```python
from build123d import *

# Parameters (mm, degrees)
F0_W     = 3
F0_H     = 15
F1_DEPTH = 16
F0_W_2   = 12
F2_DEPTH = 3
F3_R     = 5.5
F4_DEPTH = 1
F5_SIZE  = 2
F6_R     = 5
F7_R     = 0.5


with BuildPart() as f1:
    # F0 (on Top) → F1 (new body)
    with BuildSketch(Plane.XY):
        with Locations((-6, 0)):
            Rectangle(F0_W, F0_H)
    extrude(amount=F1_DEPTH)

    # F0 (on Top) → F2 (join)
    with BuildSketch(Plane.XY):
        with Locations((1.5, 0)):
            Rectangle(F0_W_2, F0_H)
        with BuildLine():
            ThreePointArc((0, -1), (-1, 0), (0, 1))
            Line((0, 1), (2, 1))
            ThreePointArc((2, 1), (2.7071067812, 0.7071067812), (3, 0))
            ThreePointArc((3, 0), (2.7071067812, -0.7071067812), (2, -1))
            Line((2, -1), (0, -1))
        make_face(mode=Mode.SUBTRACT)
    extrude(amount=F2_DEPTH)

    # F3 (on face) → F4 (cut)
    with BuildSketch(Plane(origin=(-7.5, 0, 0), x_dir=(0, -1, 0), z_dir=(-1, 0, 0))):
        with Locations((0, 8)):
            Circle(F3_R)
    extrude(amount=-F4_DEPTH, mode=Mode.SUBTRACT)

    # F5
    f5_edges = [f1.edges().sort_by_distance(p)[0] for p in [
        (-1, 0, 3),
    ]]
    chamfer(f5_edges, length=F5_SIZE)

    # F6
    f6_edges = [f1.edges().sort_by_distance(p)[0] for p in [
        (-6, -7.5, 16),
        (-6, 7.5, 16),
        (7.5, -7.5, 1.5),
        (7.5, 7.5, 1.5),
    ]]
    fillet(f6_edges, radius=F6_R)

    # F7
    f7_edges = [f1.edges().sort_by_distance(p)[0] for p in [
        (-7.5, 5.5, 8),
        (-7.5, 6.035534, 14.535534),
        (-4.5, -6.035534, 14.535534),
        (6.035534, -6.035534, 3),
    ]]
    fillet(f7_edges, radius=F7_R)


solid = f1.part
```
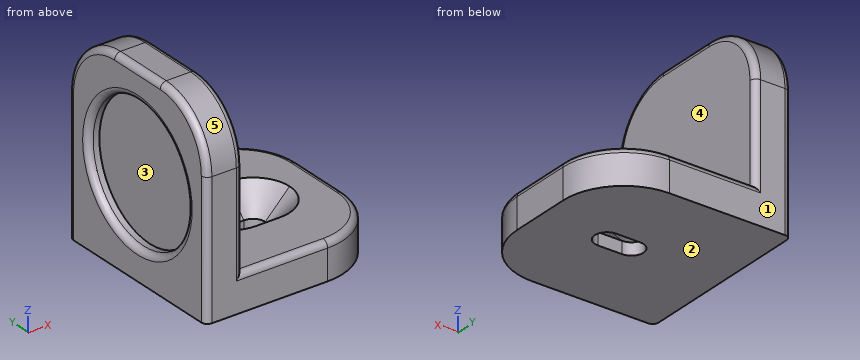
Design review of the part built by this model. Coordinates are the model's own, in mm. Face numbers are marked on the shaded views. A direction names the side the tool comes from. Coordinates: 2 decimals unless noted, no trailing zeros. Order: outer loops, then holes, each group sorted by start corner. A loop starts at its lowest first (then second) coordinate and runs counter-clockwise, first axis right, second up.
1) Take a section at A-A, the plane x = 1.25. Give the boundary of the cut face in (y, z), and give its area (3 significant figures).
2) Mouldability with a two-part tool opening along Z and no side actions: class the marked faces 1, 2 and 3 as +Z half, -Z half, draft (parallel to the pull), parting line (faces both ways), or undercut.
3) Wall thickness on line 1 along Z through (x, y) = (-6.7, 0); line 2 along Z through (x, y) = (5.5, 3.5); line 3 along X through (y, z) = (6.5, 6): over which ranges is each line inside the solid? List them lowest first.
4) For the marked faces 4 and 5, list the 3-axis set-ups (+Z, -Z, +X, -X, +Y, -Y) from which the entire face can be reached by the end or side of a thin tool; tool diameter is ignored.
5) Clearance check with flat-ended pins moving along their axes: pin 1 (4 mm diameter, centred on y = 3, z = 11.5, fed in from +X); pin 2 (6 mm diameter, centred on x = -3.5, z = 6, fed in from +Y); pin 3 (9 mm diameter, centred on x = 2.5, y = -2.5, fed in from +Z). State where each tip first meets the part, or that it passes through.
6) Take a section at B-B, the plane z = 8. Give the boundary of the cut face in (x, y).
Returned:
1. outline: (-7.5, 0) - (-1, 0) - (-1, 1) - (-3, 3) - (-7, 3) arc R0.5 ccw to (-7.5, 2.5) - close; (1, 0) - (7.5, 0) - (7.5, 2.5) arc R0.5 ccw to (7, 3) - (3, 3) - (1, 1) - close
1. area: 34.9 mm2
2. face 1: draft
2. face 2: -Z half
2. face 3: undercut
3. line 1: z = 0 to 2.5, 13.5 to 16
3. line 2: z = 0 to 3
3. line 3: x = -7.5 to -4.5
4. face 4: +Z, +X, +Y, -Y
4. face 5: +Z, +X, -X, -Y
5. pin 1: stops at x = -4.5
5. pin 2: stops at y = 7.5
5. pin 3: stops at z = 3
6. outline: (-7.5, -7) arc R0.5 ccw to (-7, -7.5) - (-5, -7.5) arc R0.5 ccw to (-4.5, -7) - (-4.5, 7) arc R0.5 ccw to (-5, 7.5) - (-7, 7.5) arc R0.5 ccw to (-7.5, 7) - (-7.5, 6) arc R0.5 ccw to (-7, 5.5) - (-6.5, 5.5) - (-6.5, -5.5) - (-7, -5.5) arc R0.5 ccw to (-7.5, -6) - close
